Here's how the part is built. I have some questions about the finished solid (model axes, mm). Face numbers are marked on the shaded views. A direction names the side the tool comes from. Coordinates: 2 decimals unless noted, no trailing zeros. Write each loop counter-clockwise with the first axis right and the second up, starting at its lowest first coordinate (ties: lowest second). Pieces come first, ordered by that corner, then holes. Notation, with made-up numbers: (19.25, -19) -> (41.25, -19) arc R26 ccw to (41.25, 16) -> close; hole circle Ø8 at (-26, 69.5). An arc over 180 degrees is marked (long way). Put each result on its own line as item: value.
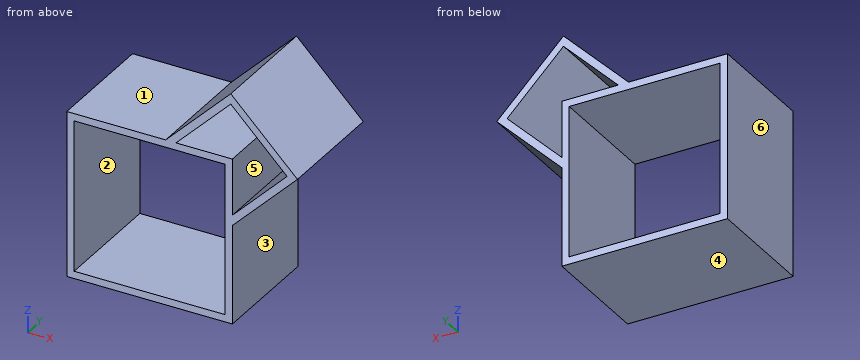
```python
from build123d import *

# Parameters (mm, degrees)
SKETCH1_W           = 71.97
SKETCH1_H           = 71.97
SKETCH1_W_2         = 65.62
SKETCH1_H_2         = 65.62
BOSS_EXTRUDE1_DEPTH = 25
BOSS_EXTRUDE2_DEPTH = 25


with BuildPart() as part:
    # Sketch1 → Boss-Extrude1 (new, symmetric)
    with BuildSketch(Plane(origin=(0, 0, 0), x_dir=(1, 0, 0), z_dir=(0, 1, 0))):
        Rectangle(SKETCH1_W, SKETCH1_H)
        Rectangle(SKETCH1_W_2, SKETCH1_H_2, mode=Mode.SUBTRACT)
    extrude(amount=BOSS_EXTRUDE1_DEPTH, both=True)

    # Sketch2 → Boss-Extrude2 (add, symmetric)
    with BuildSketch(Plane(origin=(0, 0, 0), x_dir=(1, 0, 0), z_dir=(0, 1, 0))):
        Polygon((35.277893219, -64.269271247), (6.993621971, -35.985), (11.483750032, -35.985), (35.277893219, -59.779143187), (59.779143187, -35.277893219), (35.985, -11.483750032), (35.985, -6.993621971), (64.269271247, -35.277893219), align=None)
    extrude(amount=BOSS_EXTRUDE2_DEPTH, both=True)


solid = part.part
```
Item 1: For P1, Ø2, axis at x = 0.5, y = -16.5, coming from the +Z side (3 decimals); P2, Ø12.5, axis at x = 23.5, y = -1.5, coming from the +Z side; P3, Ø5, axis at y = -8.5, z = 15, coming from the +X side, each with a flat end and sliding along its axis, tell me the tip position at first contact or that it passes through.
Output:
P1: stops at z = 35.985
P2: stops at z = 58.74
P3: stops at x = 46.49
Item 2: If we mould it in two halves opening along Z, with no side actions, what happens to the marked faces 1, 2, 3 and 4? For each: released by +Z, released by -Z, zero draft, split by the parting line, or undercut.
Output:
face 1: released by +Z
face 2: undercut
face 3: zero draft
face 4: released by -Z
Item 3: Imagine slicing it at D-D on x = 13.5. Write out the boundary of the cut face in (y, z) (3 decimals), then the cut area to 3 significant figures.
Output:
outline: (-25, -35.985) -> (25, -35.985) -> (25, -32.81) -> (-25, -32.81) -> close; (-25, 32.81) -> (25, 32.81) -> (25, 35.985) -> (-25, 35.985) -> close; (-25, 38.001) -> (25, 38.001) -> (25, 42.491) -> (-25, 42.491) -> close
area: 542 mm²
Item 4: Imagine slicing it at B-B on y = 13. Write out the boundary of the cut face in (x, z) (3 decimals).
Output:
outline: (-35.985, -35.985) -> (35.985, -35.985) -> (35.985, 6.994) -> (64.269, 35.278) -> (35.278, 64.269) -> (6.994, 35.985) -> (-35.985, 35.985) -> close; hole (-32.81, -32.81) -> (32.81, -32.81) -> (32.81, 32.81) -> (-32.81, 32.81) -> close; hole (11.484, 35.985) -> (35.985, 35.985) -> (35.985, 11.484) -> (59.779, 35.278) -> (35.278, 59.779) -> close
Item 5: Which directions (+Z, -Z, +X, -X, +Y, -Y) give clear straight access to the entire face, cutting with the end or side of a thin tool? Please do the marked faces 5 and 6.
Output:
face 5: +Y, -Y
face 6: +Z, -Z, -X, +Y, -Y
Item 6: Imagine slicing it at A-A on x = -24. Write out the boundary of the cut face in (y, z) (3 decimals).
Output:
outline: (-25, -35.985) -> (25, -35.985) -> (25, -32.81) -> (-25, -32.81) -> close; (-25, 32.81) -> (25, 32.81) -> (25, 35.985) -> (-25, 35.985) -> close
Item 7: Imagine slicing it at C-C on z = -5.5. Write out the boundary of the cut face in (x, y) (3 decimals).
Output:
outline: (-35.985, -25) -> (-32.81, -25) -> (-32.81, 25) -> (-35.985, 25) -> close; (32.81, -25) -> (35.985, -25) -> (35.985, 25) -> (32.81, 25) -> close
Item 8: Please list where these lines run through material, in increasing order: line 1 along Z through (x, y) = (-16.5, -2.5) (3 decimals); line 2 along Z through (x, y) = (24, 15) (3 decimals); line 3 along Z through (x, y) = (32, 15.5) (3 decimals). Write a range as from..to.
Output:
line 1: z = -35.985..-32.81, 32.81..35.985
line 2: z = -35.985..-32.81, 32.81..35.985, 48.501..52.991
line 3: z = -35.985..-32.81, 32.81..35.985, 56.501..60.991
